For this review, take the finished solid that the model builds, in its own axes (mm). Face numbers are marked on the shaded views. A direction names the side the tool comes from. Give positions to 0.01 mm unless a question says otherwise; leave off trailing zeros. Loops run counter-clockwise (first coordinate to the right, second up) from the corner with the lowest first, then second, coordinate; pieces in that order, holes last.
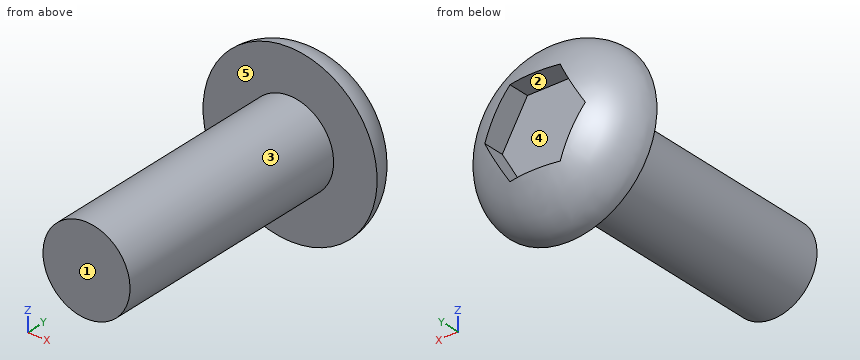
```python
from build123d import *

# Parameters (mm, degrees)
SKETCH1_R           = 2.5
BOSS_EXTRUDE1_DEPTH = 14.334
CUT_EXTRUDE1_DEPTH  = 1.778


with BuildPart() as part:
    # Sketch1 → Boss-Extrude1 (new body)
    with BuildSketch(Plane(origin=(0, 0, 0), x_dir=(1, 0, 0), z_dir=(0, 1, 0))):
        with Locations(Location((0, 0, 0), (0, 0, 270))):
            Circle(SKETCH1_R)
    extrude(amount=BOSS_EXTRUDE1_DEPTH)

    # Sketch2 → Revolve1 (revolve)
    with BuildSketch(Plane(origin=(0, 0, 0), x_dir=(0, 0, -1), z_dir=(1, 0, 0))):
        with BuildLine():
            Line((0, 14.334), (5, 14.334))
            add(Edge.make_bspline(
                [(5, 14.334), (5, 17.334), (0, 17.334)],
                knots=[0, 0, 0, 1.570796327, 1.570796327, 1.570796327], degree=2, weights=[1, 0.707106781, 1]))
            Line((0, 17.334), (0, 14.334))
        make_face()
    revolve(axis=Axis((0, 14.334, 0), (0, 1, 0)))

    # Sketch4 → Cut-Extrude1 (cut)
    with BuildSketch(Plane(origin=(0, 17.334, 0), x_dir=(1, 0, 0), z_dir=(0, 1, 0))):
        Polygon((2.886751346, 0), (1.443375673, 2.5), (-1.443375673, 2.5), (-2.886751346, 0), (-1.443375673, -2.5), (1.443375673, -2.5), align=None)
    extrude(amount=-CUT_EXTRUDE1_DEPTH, mode=Mode.SUBTRACT)


solid = part.part
```
Q1. Consider section A-A on y = 11. Give the boundary of the cut face in (x, z), plus the area to 3 significant figures.
Answers:
outline: circle Ø5 at (0, 0)
area: 19.6 mm2
Q2. For pin 1 Ø2 at (x, y) = (-3, 8.5) entering from -Z; pin 2 Ø0.7 at (x, y) = (0.5, 16.5) entering from -Z; pin 3 Ø3 at (y, z) = (7.5, -3.5) entering from -X, all flat-tipped, find the tip position at first contact; note any pin that passes through.
Answers:
pin 1: stops at z = -1.5
pin 2: stops at z = -3.95
pin 3: stops at x = -1.5
Q3. Machinability: for the marked faces 4 and 5, which of the approach directions +Z, -Z, +X, -X, +Y, -Y give a long, thin tool a straight path to every point of the face, cutting with its end or side? Answer none if there is none.
Answers:
face 4: +Y
face 5: -Y
Q4. Mouldability with a two-part tool opening along X and no side actions: class the marked faces 1, 2 and 3 as +X half, -X half, draft (parallel to the pull), parting line (faces both ways), or undercut.
Answers:
face 1: draft
face 2: undercut
face 3: parting line
Q5. For probe 1 along Y at (x, z) = (-1.5, -1.5); probe 2 along Y at (x, z) = (-3.5, 0.5); probe 3 along X at (y, z) = (6.5, 2), list the stretches that pass through material, from the lowest coordinate up.
Answers:
probe 1: y = 0 to 15.56
probe 2: y = 14.33 to 16.46
probe 3: x = -1.5 to 1.5
